Read the model definition and answer for the solid it produces. Units are mm, in the model's axes. A direction names the side the tool comes from. Coordinates: 2 decimals unless noted, no trailing zeros. Loops run counter-clockwise (first coordinate to the right, second up) from the corner with the lowest first, then second, coordinate; pieces in that order, holes last.
Q1. Straight lines are drawn through the part: line 1 (X direction, y = 0, z = 2); line 2 (Y direction, x = -8, z = 7.5); line 3 (X direction, y = -9, z = 8.75). For each, find the intervals that lie inside material, in ascending order.
Q2. Section D-D (y = 28.5) is taken. Give the vertices of the cut face in (x, z), then the cut area to 3 significant figures.
Q3. Section A-A (x = 0) is taken. Give the vertices of the cut face in (y, z), then the cut area to 3 significant figures.
Q4. Section B-B (z = 17.5) is taken. Give the vertices of the cut face in (x, y), then the cut area to 3 significant figures.
Q5. The mould has two halves that part along Y. Classify faces 3 (the face through (-1, 63.5, 9)), 4 (the face through (63.5, -1, 9)), 5 (the face through (59.68, -59.88, 9.66)), 6 (the face through (29.01, -17.063, 12.789)): pulls with the +Y half, pulls with the -Y half, needs draft (parallel to the pull), parting line crosses it, or undercut.
Q6. Section C-C (x = -17.5) is taken. Give the vertices of the cut face in (y, z), then the cut area to 3 significant figures.
Q7. A flat-ended cylindrical pin translates along its axis: P1, Ø20, axis at x = 6.5, y = 13.5, coming from the +Z side. Find the tip coordinate at first contact, or state that the pin passes through.
Q8. Which of the six approach directions +Z, -Z, +X, -X, +Y, -Y give full straight-line access (tool end or side, diameter ignored) to faces 1 (the face through (13, 1, 0)), 2 (the face through (-29.01, 17.063, 12.789))?
from build123d import *

# Parameters (mm, degrees)
F0_W     = 127
F0_H     = 127
F1_DEPTH = 19.05
F3_DEPTH = 12.7
F4_R     = 12.7
F5_R     = 12.7
F6_DEPTH = 25.4


with BuildPart() as f1:
    # F0 (on Top) → F1 (new body)
    with BuildSketch(Plane.XY):
        Rectangle(F0_W, F0_H)
    extrude(amount=F1_DEPTH)

    # F2 (on face) → F3 (cut)
    with BuildSketch(Plane.XY.offset(19.05)):
        Polygon((19.431, -33.655479), (38.862, 0), (19.431, 33.655479), (-19.431, 33.655479), (-38.862, 0), (-19.431, -33.655479), align=None)
    extrude(amount=-F3_DEPTH, mode=Mode.SUBTRACT)

    # F4
    f4_edges = [f1.edges().sort_by_distance(p)[0] for p in [
        (-63.5, -63.5, 9.525),
        (63.5, -63.5, 9.525),
        (63.5, 63.5, 9.525),
        (-63.5, 63.5, 9.525),
    ]]
    fillet(f4_edges, radius=F4_R)

    # F5 (on face) → F6 (cut)
    with BuildSketch(Plane(origin=(0, 0, 0), x_dir=(1, 0, 0), z_dir=(0, 0, -1))):
        Circle(F5_R)
    extrude(amount=-F6_DEPTH, mode=Mode.SUBTRACT)


solid = f1.part
Numbers:
1. line 1: x = -63.5 to -12.7, 12.7 to 63.5
1. line 2: y = -63.5 to -33.66, 33.66 to 63.5
1. line 3: x = -63.5 to -33.67, 33.67 to 63.5
2. outline: (-63.5, 0) - (63.5, 0) - (63.5, 19.05) - (22.41, 19.05) - (22.41, 6.35) - (-22.41, 6.35) - (-22.41, 19.05) - (-63.5, 19.05) - close
2. area: 1,850 mm2
3. outline: (-63.5, 0) - (-12.7, 0) - (-12.7, 6.35) - (-33.66, 6.35) - (-33.66, 19.05) - (-63.5, 19.05) - close; (12.7, 0) - (63.5, 0) - (63.5, 19.05) - (33.66, 19.05) - (33.66, 6.35) - (12.7, 6.35) - close
3. area: 1,400 mm2
4. outline: (-63.5, -50.8) arc R12.7 ccw to (-50.8, -63.5) - (50.8, -63.5) arc R12.7 ccw to (63.5, -50.8) - (63.5, 50.8) arc R12.7 ccw to (50.8, 63.5) - (-50.8, 63.5) arc R12.7 ccw to (-63.5, 50.8) - close; hole (-38.86, 0) - (-19.43, -33.66) - (19.43, -33.66) - (38.86, 0) - (19.43, 33.66) - (-19.43, 33.66) - close
4. area: 12,100 mm2
5. face 3: pulls with the +Y half
5. face 4: needs draft
5. face 5: pulls with the -Y half
5. face 6: undercut
6. outline: (-63.5, 0) - (63.5, 0) - (63.5, 19.05) - (33.66, 19.05) - (33.66, 6.35) - (-33.66, 6.35) - (-33.66, 19.05) - (-63.5, 19.05) - close
6. area: 1,560 mm2
7. P1: stops at z = 6.35
8. face 1: -Z, +X, -X, +Y, -Y
8. face 2: +Z
